The listing builds one solid part. Answer for the finished solid, in the listing's coordinates (mm). A direction names the side the tool comes from. Coordinates: 2 decimals unless noted, no trailing zeros. Loops run counter-clockwise (first coordinate to the right, second up) from the corner with the lowest first, then second, coordinate; pieces in that order, holes last. Notation, with made-up numbers: (49.25, -2.75) - (58.25, -2.75) arc R20 ccw to (58.25, 14.25) - close; hole circle Ø10 at (-30.75, -4). An arc over 180 degrees is marked (long way). Put each result on its own line as item: value.
```python
from build123d import *

# Parameters (mm, degrees)
F0_W     = 20.32
F0_H     = 20.32
F1_DEPTH = 2.921
F3_D     = 2.54
F5_R     = 2.54
F4_W     = 17.78
F4_H     = 2.54
F6_DEPTH = 5.334
F8_D     = 1.27


# Not quite as in the source:
# - a pattern or mirror of a feature is missing from the dataset's text; its kind, count and spacing are read off the source's solid


with BuildPart() as f1:
    # F0 (on Top) → F1 (new body)
    with BuildSketch(Plane.XY):
        Rectangle(F0_W, F0_H)
    extrude(amount=F1_DEPTH)

    # F3 (through all)
    with Locations(Plane.XY.offset(2.921)):
        with Locations((-7.62, 7.2416714393)):
            f3 = Hole(F3_D / 2)

    # F3_copies: F3 across plane
    add(f3.mirror(Plane(origin=(0, 0, 0), x_dir=(0, 0, 1), z_dir=(1, 0, 0))), mode=Mode.SUBTRACT)

    # F5
    f5_edges = [f1.edges().sort_by_distance(p)[0] for p in [
        (-10.16, 10.16, 1.4605),
        (10.16, 10.16, 1.4605),
        (-10.16, -10.16, 1.4605),
        (10.16, -10.16, 1.4605),
    ]]
    fillet(f5_edges, radius=F5_R)

    # F4 (on face) → F6 (join)
    with BuildSketch(Plane.XY.offset(2.921)):
        with Locations((0, -7.366)):
            Rectangle(F4_W, F4_H)
    extrude(amount=F6_DEPTH)

    # F8 (through all)
    with Locations(Plane.XY.offset(2.921)):
        with Locations((0, 0)):
            Hole(F8_D / 2)


solid = f1.part
```
1) The part is cut by section C-C (z = 6.25). Give the vertices of the cut face in (x, y).
Found:
outline: (-8.89, -8.64) - (8.89, -8.64) - (8.89, -6.1) - (-8.89, -6.1) - close
2) Straight lines are drawn through the part: L1, parallel to Y at x = 0, z = 2.05 (3 decimals); L2, parallel to Z at x = -5.5, y = 8.5; L3, parallel to X at y = -6.75, z = 5.75. For each, find the intervals that lie inside material, in ascending order. Write a range as [from, to].
Found:
L1: y = [-10.16, -0.635], [0.635, 10.16]
L2: z = [0, 2.92]
L3: x = [-8.89, 8.89]
3) For faces 1 (the face through (0, -6.096, 6)), 2 (the face through (-8.89, -7, 6)), 3 (the face through (8.89, -7, 6)), determine the directions among +Z, -Z, +X, -X, +Y, -Y from which every point of the face is accessible in a straight line to the end or side of a thin tool.
Found:
face 1: +Z, +X, -X, +Y
face 2: +Z, -X, +Y, -Y
face 3: +Z, +X, +Y, -Y
4) The part is cut by section D-D (y = 5.25). Give the vertices of the cut face in (x, z).
Found:
outline: (-10.16, 0) - (10.16, 0) - (10.16, 2.92) - (-10.16, 2.92) - close
5) For a pull along Y with two mould halves and no side action, classify faces 4 (the face through (-8.793, 6.755, 1.44)), 5 (the face through (8.206, 6.115, 1.44)), 6 (the face through (-10.16, 0, 1)), 7 (the face through (0, -10.16, 1)) as pulls with the +Y half, pulls with the -Y half, needs draft (parallel to the pull), parting line crosses it, or undercut.
Found:
face 4: undercut
face 5: undercut
face 6: needs draft
face 7: pulls with the -Y half
6) Each of these flat-tipped pins is pushed along its axis until it touches: pin 1 (2 mm diameter, centred on y = -7, z = 3, fed in from +X); pin 2 (2 mm diameter, centred on y = -7.5, z = 4.5, fed in from -X); pin 3 (3 mm diameter, centred on x = -1.5, y = 2, fed in from +Z); pin 4 (1.6 mm diameter, centred on x = -3, z = 5, fed in from +Y). Where does it stop, or does it pass through?
Found:
pin 1: stops at x = 10.16
pin 2: stops at x = -8.89
pin 3: stops at z = 2.92
pin 4: stops at y = -6.1
7) The part is cut by section A-A (x = 0). Give the vertices of the cut face in (y, z) (3 decimals), and give its area (3 significant figures).
Found:
outline: (-10.16, 0) - (-0.635, 0) - (-0.635, 2.921) - (-6.096, 2.921) - (-6.096, 8.255) - (-8.636, 8.255) - (-8.636, 2.921) - (-10.16, 2.921) - close; (0.635, 0) - (10.16, 0) - (10.16, 2.921) - (0.635, 2.921) - close
area: 69.2 mm^2
8) The part is cut by section B-B (y = 0). Give the vertices of the cut face in (x, z) (3 decimals), and give its area (3 significant figures).
Found:
outline: (-10.16, 0) - (-0.635, 0) - (-0.635, 2.921) - (-10.16, 2.921) - close; (0.635, 0) - (10.16, 0) - (10.16, 2.921) - (0.635, 2.921) - close
area: 55.6 mm^2
